Read the model definition and answer for the solid it produces. Units are mm, in the model's axes. A direction names the side the tool comes from. Coordinates: 2 decimals unless noted, no trailing zeros. Loops run counter-clockwise (first coordinate to the right, second up) from the corner with the lowest first, then second, coordinate; pieces in that order, holes last. Notation, with made-up numbers: (39.25, -2) - (75.25, -2) arc R17 cw to (75.25, 25) - close; hole circle Ø2 at (35.5, 66). An arc over 180 degrees is marked (long way). Use one line per item in the form item = value. Start each with the question number.
1) Consider line 1 (X direction, y = -10.5, z = -4); line 2 (X direction, y = -22.5, z = 17); line 3 (Z direction, x = -58, y = -3). Determine where each line is inside the solid, lowest interval first.
2) A cutting plane is placed at B-B (z = 30). Give the vertices of the cut face in (x, y), and give its area (3 significant figures).
3) The mould has two halves that part along Z. Classify faces 4 (the face through (-85.39, -12.52, 31.99)), 5 (the face through (-98.63, -12.52, 14.26)), 6 (the face through (-35.941, -13, -3)): released by +Z, released by -Z, zero draft, split by the parting line, or undercut.
4) A cutting plane is placed at C-C (x = -1.5). Give the vertices of the cut face in (y, z), and give its area (3 significant figures).
5) A cutting plane is placed at A-A (y = -4.5). Give the vertices of the cut face in (x, z).
6) Which of the six approach directions +Z, -Z, +X, -X, +Y, -Y give full straight-line access (tool end or side, diameter ignored) to faces 1 (the face through (-51, -13, -17.952)), 2 (the face through (-79, -13, 42.165)), 3 (the face through (-7, 0, 20))?
7) Each of these flat-tipped pins is pushed along its axis until it touches: P1, Ø6, axis at x = -61, y = -19, coming from the +Z side; P2, Ø3, axis at x = 12, y = -10.5, coming from the +Z side; P3, Ø1.5, axis at x = 66, y = -11, coming from the +Z side. Where does it stop, or does it pass through?
8) A cutting plane is placed at D-D (z = -2). Give the vertices of the cut face in (x, y).
from build123d import *

# Parameters (mm, degrees)
F0_R     = 6.58625
F1_DEPTH = 21.082
F2_DEPTH = 25.4
F3_SIZE  = 5.08


with BuildPart() as f1:
    # F0 (on Front) → F1 (new body)
    with BuildSketch(Plane.XZ):
        with BuildLine():
            Line((91.058975, 12.527699), (91.058975, 43.007699))
            Line((91.058975, 43.007699), (-57.654542, 42.165341))
            Line((-57.654542, 42.165341), (-101.388322, 42.165341))
            Line((-101.388322, 42.165341), (-101.113739, 11.686578))
            Line((-101.113739, 11.686578), (-68.093739, 11.686578))
            ThreePointArc((-68.093739, 11.686578), (-82.944012, -4.153037), (-66.180828, -17.952301))
            Line((-66.180828, -17.952301), (-35.941025, -17.952301))
            Line((-35.941025, -17.952301), (-35.941025, 12.527699))
            Line((-35.941025, 12.527699), (91.058975, 12.527699))
        make_face()
        with Locations((-88.930964, 26.435958)):
            Circle(F0_R, mode=Mode.SUBTRACT)
    extrude(amount=F1_DEPTH)

    # F0 (on Front) → F2 (join)
    with BuildSketch(Plane.XZ):
        with BuildLine():
            Line((91.058975, 12.527699), (91.058975, 43.007699))
            Line((91.058975, 43.007699), (-57.654542, 42.165341))
            Line((-57.654542, 42.165341), (-101.388322, 42.165341))
            Line((-101.388322, 42.165341), (-101.113739, 11.686578))
            Line((-101.113739, 11.686578), (-68.093739, 11.686578))
            ThreePointArc((-68.093739, 11.686578), (-82.944012, -4.153037), (-66.180828, -17.952301))
            Line((-66.180828, -17.952301), (-35.941025, -17.952301))
            Line((-35.941025, -17.952301), (-35.941025, 12.527699))
            Line((-35.941025, 12.527699), (91.058975, 12.527699))
        make_face()
        with Locations((-88.930964, 26.435958)):
            Circle(F0_R, mode=Mode.SUBTRACT)
    extrude(amount=F2_DEPTH)

    # F3
    f3_edges = [f1.edges().sort_by_distance(p)[0] for p in [
        (-101.113739, -12.7, 11.686578),
    ]]
    chamfer(f3_edges, length=F3_SIZE)


solid = f1.part
Found:
q1.line_1 = -82.95 to -35.94
q1.line_2 = -101.16 to 91.06
q1.line_3 = -17.95 to 42.17
q2.outline = (-101.28, -25.4) - (-94.47, -25.4) - (-94.47, 0) - (-101.28, 0) - close; (-83.39, -25.4) - (91.06, -25.4) - (91.06, 0) - (-83.39, 0) - close
q2.area = 4,600 mm^2
q3.face_4 = undercut
q3.face_5 = released by -Z
q3.face_6 = zero draft
q4.outline = (-25.4, 12.53) - (0, 12.53) - (0, 42.48) - (-25.4, 42.48) - close
q4.area = 761 mm^2
q5.outline = (-101.39, 42.17) - (-101.16, 16.77) - (-96.03, 11.69) - (-68.09, 11.69) arc R14.88 ccw (long way) to (-66.18, -17.95) - (-35.94, -17.95) - (-35.94, 12.53) - (91.06, 12.53) - (91.06, 43.01) - (-57.65, 42.17) - close; hole circle Ø13.17 at (-88.93, 26.44)
q6.face_1 = -Z, +X, +Y, -Y
q6.face_2 = +Z, -X, +Y, -Y
q6.face_3 = +Z, -Z, +X, -X, +Y
q7.P1 = 42.17
q7.P2 = 42.57
q7.P3 = 42.87
q8.outline = (-82.93, -25.4) - (-35.94, -25.4) - (-35.94, 0) - (-82.93, 0) - close
